```python
from build123d import *

# Parameters (mm, degrees)
F1_DEPTH = 6.35
F2_R     = 1.27


with BuildPart() as f1:
    # F0 (on Front) → F1 (new body)
    with BuildSketch(Plane.XZ):
        with BuildLine():
            ThreePointArc((-69.85, 25.4), (-70.1243474386, 22.1786073053), (-70.9394877579, 19.05))
            Line((-70.9394877579, 19.05), (70.9394877579, 19.05))
            ThreePointArc((70.9394877579, 19.05), (70.1243474386, 22.1786073053), (69.85, 25.4))
            Line((69.85, 25.4), (-69.85, 25.4))
        make_face()
        with BuildLine():
            Line((-88.9, 12.7), (-88.9, 6.35))
            ThreePointArc((-88.9, 6.35), (-85.6786055668, 6.6243477369), (-82.5499966741, 7.4394889338))
            ThreePointArc((-82.5499966741, 7.4394889338), (-75.4296145712, 11.9296170656), (-70.9394877579, 19.05))
            ThreePointArc((-70.9394877579, 19.05), (-70.1243474386, 22.1786073053), (-69.85, 25.4))
            Line((-69.85, 25.4), (-76.2, 25.4))
            ThreePointArc((-76.2, 25.4), (-79.9197438789, 16.4197438789), (-88.9, 12.7))
        make_face()
        with BuildLine():
            ThreePointArc((-88.9, -12.7), (-79.9197438789, -16.4197438789), (-76.2, -25.4))
            Line((-76.2, -25.4), (-69.85, -25.4))
            ThreePointArc((-69.85, -25.4), (-70.1243475845, -22.1786064547), (-70.9394883332, -19.0499983728))
            ThreePointArc((-70.9394883332, -19.0499983728), (-75.4296151814, -11.9296164554), (-82.5499966741, -7.4394889338))
            ThreePointArc((-82.5499966741, -7.4394889338), (-85.6786055668, -6.6243477369), (-88.9, -6.35))
            Line((-88.9, -6.35), (-88.9, -12.7))
        make_face()
        with BuildLine():
            Line((-88.9, 6.35), (-88.9, -6.35))
            ThreePointArc((-88.9, -6.35), (-85.6786055668, -6.6243477369), (-82.5499966741, -7.4394889338))
            Line((-82.5499966741, -7.4394889338), (-82.5499966741, 7.4394889338))
            ThreePointArc((-82.5499966741, 7.4394889338), (-85.6786055668, 6.6243477369), (-88.9, 6.35))
        make_face()
        with BuildLine():
            ThreePointArc((-70.9394883332, -19.0499983728), (-70.1243475845, -22.1786064547), (-69.85, -25.4))
            Line((-69.85, -25.4), (69.85, -25.4))
            ThreePointArc((69.85, -25.4), (70.1243475845, -22.1786064547), (70.9394883332, -19.0499983728))
            Line((70.9394883332, -19.0499983728), (-70.9394883332, -19.0499983728))
        make_face()
        with BuildLine():
            ThreePointArc((70.9394883332, -19.0499983728), (70.1243475845, -22.1786064547), (69.85, -25.4))
            Line((69.85, -25.4), (76.2, -25.4))
            ThreePointArc((76.2, -25.4), (79.9197438789, -16.4197438789), (88.9, -12.7))
            Line((88.9, -12.7), (88.9, -6.35))
            ThreePointArc((88.9, -6.35), (85.6786073053, -6.6243474386), (82.55, -7.4394877579))
            ThreePointArc((82.55, -7.4394877579), (75.4296164286, -11.9296152082), (70.9394883332, -19.0499983728))
        make_face()
        with BuildLine():
            Line((82.55, 7.4394877579), (82.55, -7.4394877579))
            ThreePointArc((82.55, -7.4394877579), (85.6786073053, -6.6243474386), (88.9, -6.35))
            Line((88.9, -6.35), (88.9, 6.35))
            ThreePointArc((88.9, 6.35), (85.6786073053, 6.6243474386), (82.55, 7.4394877579))
        make_face()
        with BuildLine():
            ThreePointArc((70.9394877579, 19.05), (75.4296158184, 11.9296158184), (82.55, 7.4394877579))
            ThreePointArc((82.55, 7.4394877579), (85.6786073053, 6.6243474386), (88.9, 6.35))
            Line((88.9, 6.35), (88.9, 12.7))
            ThreePointArc((88.9, 12.7), (79.9197438789, 16.4197438789), (76.2, 25.4))
            Line((76.2, 25.4), (69.85, 25.4))
            ThreePointArc((69.85, 25.4), (70.1243474386, 22.1786073053), (70.9394877579, 19.05))
        make_face()
    extrude(amount=F1_DEPTH)

    # F2
    f2_edges = [f1.edges().sort_by_distance(p)[0] for p in [
        (-79.919744, -6.35, 16.419744),
        (-88.9, -6.35, 0),
        (-79.919744, -6.35, -16.419744),
        (0, -6.35, -25.4),
        (0, -6.35, 25.4),
        (79.919744, -6.35, 16.419744),
        (88.9, -6.35, 0),
        (79.919744, -6.35, -16.419744),
        (82.55, -6.35, 0),
        (75.429616, -6.35, 11.929616),
        (0, -6.35, 19.05),
        (-75.429615, -6.35, 11.929617),
        (-82.549997, -6.35, 0),
        (-75.429615, -6.35, -11.929616),
        (0, -6.35, -19.049998),
        (75.429616, -6.35, -11.929615),
    ]]
    fillet(f2_edges, radius=F2_R)


solid = f1.part
```
Geometry: final body of the model. Coordinates: model frame, mm. A direction names the side the tool comes from. Coordinates: 2 decimals unless noted, no trailing zeros. Loops run counter-clockwise (first coordinate to the right, second up) from the corner with the lowest first, then second, coordinate; pieces in that order, holes last. Notation, with made-up numbers: M 79,-28.75 L 116,-28.75 A15 ccw 116,-12.75 Z; hole C -14.75,49.25 d10. An arc over 180 degrees is marked long. Put each result on its own line as item: value.
(1) Material intervals for probe 1 along X at (y, z) = (-0.75, 1.5); probe 2 along Z at (x, y) = (50.5, -4.75); probe 3 along Z at (x, y) = (-21, -5.25), sorted ascending.
Answer sheet:
probe 1: x = -88.9 to -82.55, 82.55 to 88.9
probe 2: z = -25.4 to -19.05, 19.05 to 25.4
probe 3: z = -25.39 to -19.06, 19.06 to 25.39
(2) Access query for faces 4 (the face through (-1, -3, 19.05)), 5 (the face through (-80.02, -2.5, -16.32)). Directions: +Z, -Z, +X, -X, +Y, -Y. A direction counts if a zero-diameter tool reaches every point of the face in a straight line with its end or side. Return the directions, or none.
Answer sheet:
face 4: +Y, -Y
face 5: -Z, -X, +Y, -Y
(3) Cut plane A-A on z = -2.5. Return the cut outline in (x, y).
Answer sheet:
outline: M -88.9,-5.08 A1.27 ccw -87.63,-6.35 L -83.82,-6.35 A1.27 ccw -82.55,-5.08 L -82.55,0 L -88.9,0 Z; M 82.55,-5.08 A1.27 ccw 83.82,-6.35 L 87.63,-6.35 A1.27 ccw 88.9,-5.08 L 88.9,0 L 82.55,0 Z
(4) Cut plane C-C on y = -3. Return the cut outline in (x, z).
Answer sheet:
outline: M -88.9,-12.7 A12.7 cw -76.2,-25.4 L 76.2,-25.4 A12.7 cw 88.9,-12.7 L 88.9,12.7 A12.7 cw 76.2,25.4 L -76.2,25.4 A12.7 cw -88.9,12.7 Z; hole M -82.55,-7.44 A19.05 cw -70.94,-19.05 L 70.94,-19.05 A19.05 cw 82.55,-7.44 L 82.55,7.44 A19.05 cw 70.94,19.05 L -70.94,19.05 A19.05 cw -82.55,7.44 Z
(5) Cut plane B-B on x = -10. Return the cut outline in (y, z).
Answer sheet:
outline: M -6.35,-24.13 A1.27 ccw -5.08,-25.4 L 0,-25.4 L 0,-19.05 L -5.08,-19.05 A1.27 ccw -6.35,-20.32 Z; M -6.35,20.32 A1.27 ccw -5.08,19.05 L 0,19.05 L 0,25.4 L -5.08,25.4 A1.27 ccw -6.35,24.13 Z
(6) Draft query along X for faces 1 (the face through (80.02, -2.5, 16.32)), 2 (the face through (-79.82, -2.5, 16.52)), 3 (the face through (75.35, -2.5, 12.01)). Return one class per face: pulls with the +X half, pulls with the -X half, needs draft (parallel to the pull), parting line crosses it, or undercut.
Answer sheet:
face 1: pulls with the +X half
face 2: pulls with the -X half
face 3: undercut
